from build123d import *

# Parameters (mm, degrees)
F1_DEPTH = 15


with BuildPart() as f1:
    # F0 (on Front) → F1 (new body)
    with BuildSketch(Plane.XZ):
        with BuildLine():
            Line((10, -15), (10, 0))
            ThreePointArc((10, 0), (0, 10), (-10, 0))
            Line((-10, 0), (-10, -15))
            Line((-10, -15), (-8.5, -15))
            Line((-8.5, -15), (-8.5, 0))
            ThreePointArc((-8.5, 0), (0, 8.5), (8.5, 0))
            Line((8.5, 0), (8.5, -15))
            Line((8.5, -15), (10, -15))
        make_face()
    extrude(amount=F1_DEPTH)


solid = f1.part
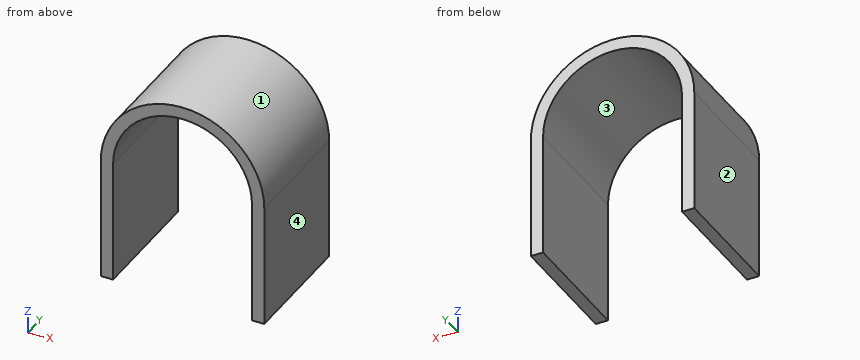
Geometry: final body of the model. Coordinates: model frame, mm. Face numbers are marked on the shaded views. Coordinates: 2 decimals unless noted, no trailing zeros. Order: outer loops, then holes, each group sorted by start corner. A loop starts at its lowest first (then second) coordinate and runs counter-clockwise, first axis right, second up. Notation, with made-up numbers: M 36.25,-12.75 L 84.25,-12.75 A23 cw 84.25,20.25 Z; hole C 88.5,-21 d4. An arc over 180 degrees is marked long. One line per question, with ' | ' between items. Start each with the question number.
Item 1: Ray query, probe 1 along X at (y, z) = (-5.5, -9.75); probe 2 along X at (y, z) = (-9.5, 6.75); probe 3 along Z at (x, y) = (7.5, -1.5). Return the intervals inside material, ascending. Write a range as [from, to].
Item 2: Cut plane B-B, the plane y = -10. Return the cut outline in (x, z), then the cut area to 3 significant figures.
Item 3: Cut plane C-C, the plane z = 3.75. Return the cut outline in (x, y), then the cut area to 3 significant figures.
Item 4: Pin query (flat end, axial travel): pin 1 Ø3 at (x, y) = (3, -7) entering from -Z; pin 2 Ø2 at (x, y) = (8, -2.5) entering from -Z; pin 3 Ø2 at (y, z) = (-7.5, 6.5) entering from +X; pin 4 Ø5 at (x, y) = (2.5, -2.5) entering from -Z. Return the tip coordinate at first contact, or that it passes through.
Item 5: Draft query along X for the marked faces 1, 2, 3 and 4. Return one class per face: released by +X, released by -X, zero draft, split by the parting line, or undercut.
Item 6: Cut plane A-A, the plane z = -9. Return the cut outline in (x, y), then the cut area to 3 significant figures.
Item 7: Cut plane D-D, the plane x = 0. Return the cut outline in (y, z), then the cut area to 3 significant figures.
A:
1) probe 1: x = [-10, -8.5], [8.5, 10] | probe 2: x = [-7.38, -5.17], [5.17, 7.38] | probe 3: z = [4, 6.61]
2) outline: M -10,-15 L -8.5,-15 L -8.5,0 A8.5 cw 8.5,0 L 8.5,-15 L 10,-15 L 10,0 A10 ccw -10,0 Z | area: 88.6 mm2
3) outline: M -9.27,-15 L -7.63,-15 L -7.63,0 L -9.27,0 Z; M 7.63,-15 L 9.27,-15 L 9.27,0 L 7.63,0 Z | area: 49.3 mm2
4) pin 1: stops at z = 7.21 | pin 2: stops at z = -15 | pin 3: stops at x = 8.35 | pin 4: stops at z = 6.87
5) face 1: split by the parting line | face 2: released by -X | face 3: undercut | face 4: released by +X
6) outline: M -10,-15 L -8.5,-15 L -8.5,0 L -10,0 Z; M 8.5,-15 L 10,-15 L 10,0 L 8.5,0 Z | area: 45.0 mm2
7) outline: M -15,8.5 L 0,8.5 L 0,10 L -15,10 Z | area: 22.5 mm2
